Geometry check sheet. Reference: the model listing, model coordinates, mm. Give positions to 0.01 mm unless a question says otherwise; leave off trailing zeros. Write each loop counter-clockwise with the first axis right and the second up, starting at its lowest first coordinate (ties: lowest second). Pieces come first, ordered by that corner, then holes. Notation, with made-up numbers: (72.5, -28) - (103.5, -28) arc R17 ccw to (103.5, -24) - close; hole circle Ø4 at (67.25, 46). An arc over 180 degrees is marked (long way). Write item = value, one per line. Start each with the question number.
(1) Section check D-D, the plane y = 20.5. Enter the section's corners in (x, z).
(2) Section check B-B, the plane z = -62.3. Enter the section's corners in (x, y), plus the area to 3 significant figures.
(3) Section check A-A, the plane y = 11.4. Enter the section's corners in (x, z).
(4) Thickness scan on L1, parallel to Z at x = 0.4, y = 11.25; L2, parallel to Y at x = 0.5, z = -62.3; L3, parallel to Z at x = 0.3, y = 1.5. Record the ranges inside material, lowest first.
(5) Section check C-C, the plane x = 0.9. Enter the section's corners in (y, z).
(6) Depth check by flat-ended pin: pin 1 Ø2 at (y, z) = (11.4, -62.3) entering from -X; pin 2 Ø0.6 at (x, y) = (0.5, 12.5) entering from +Z. Enter the tip coordinate at first touch or a pass-through.
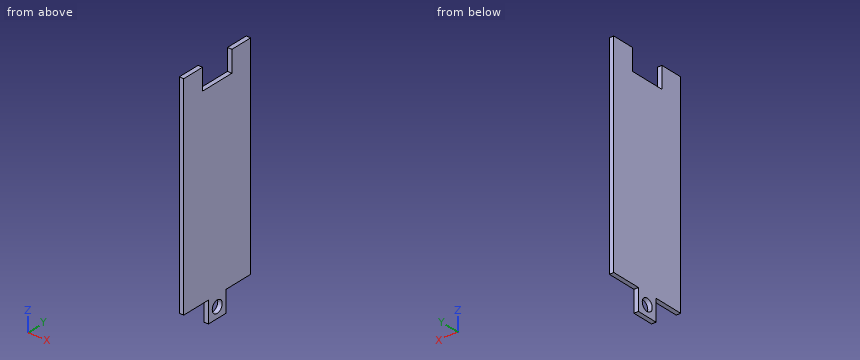
Autodesk Inventor part; units mm, degrees
ref_plane "YZ Plane" through (0, 0, 0) normal (1, 0, 0) x (0, 1, 0)
ref_plane "XZ Plane" through (0, 0, 0) normal (0, 1, 0) x (-1, 0, 0)
ref_plane "XY Plane" through (0, 0, 0) normal (0, 0, 1) x (1, 0, 0)
sketch "Sketch1" plane through (0, 0, 0) normal (1, 0, 0) x (0, 1, 0)
  line L0 (0, 0) -> (0, -59.3)
  line L1 (0, -59.3) -> (22.8, -59.3)
  line L2 (22.8, -59.3) -> (22.8, 0)
  line L3 (22.8, 0) -> (0, 0)
  dimension "d0" = 59.3
  dimension "d1" = 22.8
extrude "Extrusion1" add sketch "Sketch1" along normal blind 1.25
sketch "Sketch2" plane through (0, 0, 0) normal (0, 0, 1) x (1, 0, 0)
  line L0 (0, 22.8) -> (0, 0)
  line L1 (0, 0) -> (1.25, 0)
  line L2 (1.25, 22.8) -> (1.25, 0)
  line L3 (0, 22.8) -> (1.25, 22.8)
  line L4 (1.25, 0) -> (1.25, 22.8)
  line L5 (1.25, 22.8) -> (1.25, 11.4)
  line L6 (1.25, 11.4) -> (1.25, 16.4)
  line L7 (1.25, 16.4) -> (0, 16.4)
  line L8 (0, 0) -> (0, 22.8)
  line L9 (0, 16.4) -> (0, 6.4)
  line L10 (0, 6.4) -> (1.25, 6.4)
  dimension "d4" = 11.4
  dimension "d5" = 5
  dimension "d6" = 10
extrude "Extrusion2" cut sketch "Sketch2" against normal blind 6 contours L7 L2 L10 L0
sketch "Sketch3" plane through (1.25, 0, 0) normal (1, 0, 0) x (0, 0, -1)
  line L0 (6, 6.4) -> (0, 6.4)
  line L1 (0, 6.4) -> (0, 0)
  line L2 (0, 0) -> (59.3, 0)
  line L3 (59.3, 0) -> (59.3, 22.8)
  line L4 (59.3, 22.8) -> (0, 22.8)
  line L5 (0, 22.8) -> (0, 16.4)
  line L6 (0, 16.4) -> (6, 16.4)
  line L7 (6, 16.4) -> (6, 6.4)
  line L8 (59.3, 0) -> (59.3, 22.8)
  line L9 (59.3, 0) -> (59.3, 11.4)
  line L10 (59.3, 11.4) -> (59.3, 8.4)
  line L11 (59.3, 8.4) -> (65.3, 8.4)
  line L12 (65.3, 8.4) -> (65.3, 14.4)
  line L13 (65.3, 14.4) -> (59.3, 14.4)
  line L14 (59.3, 11.4) -> (62.3, 11.4)
  circle A0 centre (62.3, 11.4) radius 1.7
  dimension "d9" = 11.4
  dimension "d10" = 3
  dimension "d11" = 6
  dimension "d12" = 6
  dimension "d13" = 3.4
extrude "Extrusion3" add sketch "Sketch3" against normal blind 1.25 contours L3 L13 L12 L11
properties part number "tapa_carcasa"
Model answer:
q1.outline = (0, -59.3) - (1.25, -59.3) - (1.25, 0) - (0, 0) - close
q2.outline = (0, 8.4) - (1.25, 8.4) - (1.25, 9.7) - (0, 9.7) - close; (0, 13.1) - (1.25, 13.1) - (1.25, 14.4) - (0, 14.4) - close
q2.area = 3.25 mm²
q3.outline = (0, -65.3) - (1.25, -65.3) - (1.25, -64) - (0, -64) - close; (0, -60.6) - (1.25, -60.6) - (1.25, -6) - (0, -6) - close
q4.L1 = -65.3 to -63.99, -60.61 to -6
q4.L2 = 8.4 to 9.7, 13.1 to 14.4
q4.L3 = -59.3 to 0
q5.outline = (0, -59.3) - (8.4, -59.3) - (8.4, -65.3) - (14.4, -65.3) - (14.4, -59.3) - (22.8, -59.3) - (22.8, 0) - (16.4, 0) - (16.4, -6) - (6.4, -6) - (6.4, 0) - (0, 0) - close; hole circle Ø3.4 at (11.4, -62.3)
q6.pin_1 = through
q6.pin_2 = -6
